Build history of the part. All positions in model axes, mm. Round coordinates to 2 decimals unless told otherwise and drop trailing zeros. Loops run counter-clockwise (first coordinate to the right, second up) from the corner with the lowest first, then second, coordinate; pieces in that order, holes last.
from build123d import *

# Parameters (mm, degrees)
SKETCH1_R           = 2.5
BOSS_EXTRUDE1_DEPTH = 20
SKETCH2_R           = 1.5
CUT_EXTRUDE1_DEPTH  = 5
FILLET1_R           = 0.5


with BuildPart() as part:
    # Sketch1 → Boss-Extrude1 (new body)
    with BuildSketch(Plane(origin=(0, 0, 0), x_dir=(1, 0, 0), z_dir=(0, 1, 0))):
        Circle(SKETCH1_R)
    extrude(amount=BOSS_EXTRUDE1_DEPTH)

    # Sketch2 → Cut-Extrude1 (cut, symmetric)
    with BuildSketch(Plane(origin=(0, 0, 0), x_dir=(0, 0, -1), z_dir=(1, 0, 0))):
        with Locations((0, 17.5)):
            Circle(SKETCH2_R)
        with Locations((0, 2.5)):
            Circle(SKETCH2_R)
    extrude(amount=CUT_EXTRUDE1_DEPTH, both=True, mode=Mode.SUBTRACT)

    # Fillet1
    fillet1_edges = [part.edges().sort_by_distance(p)[0] for p in [
        (-2.5, 0, 0),
        (-2.5, 20, 0),
    ]]
    fillet(fillet1_edges, radius=FILLET1_R)


solid = part.part
(1) Pull direction Z, two halves, no side cores. Call faces 1 (the face through (-2.5, 9.9, -0.1)), 2 (the face through (0.03, 2.57, 1.5)), 3 (the face through (0, 20, 0)): +Z half, -Z half, draft (parallel to the pull), parting line (faces both ways), or undercut.
Responses:
face 1: parting line
face 2: undercut
face 3: draft
(2) Slice it at A-A on z = 0. List the corners of the cut face in (x, y), plus the area to 3 significant figures.
Responses:
outline: (-2.5, 0.5) arc R0.5 ccw to (-2, 0) - (2, 0) arc R0.5 ccw to (2.5, 0.5) - (2.5, 1) - (-2.5, 1) - close; (-2.5, 4) - (2.5, 4) - (2.5, 16) - (-2.5, 16) - close; (-2.5, 19) - (2.5, 19) - (2.5, 19.5) arc R0.5 ccw to (2, 20) - (-2, 20) arc R0.5 ccw to (-2.5, 19.5) - close
area: 69.8 mm2
(3) Pin check, flat tips, straight feed: P1, Ø2, axis at y = 10.5, z = -2, coming from the -X side; P2, Ø2, axis at y = 3, z = -0.5, coming from the -X side. Stop position of each tip, or through.
Responses:
P1: stops at x = -2.29
P2: stops at x = -2.48
(4) Probe line 1 (Y direction, x = -0.75, z = 0); line 2 (Y direction, x = -2, z = 0.55); line 3 (X direction, y = 4.5, z = 1.5). List the from-to ranges inside material, lowest first.
Responses:
line 1: y = 0 to 1, 4 to 16, 19 to 20
line 2: y = 0.01 to 1.1, 3.9 to 16.1, 18.9 to 19.99
line 3: x = -2 to 2
(5) Slice it at C-C on y = 12.75. List the corners of the cut face in (x, z), plus the area to 3 significant figures.
Responses:
outline: circle Ø5 at (0, 0)
area: 19.6 mm2
(6) Slice it at D-D on x = 0.6. Count the separate pieces of the cut face and the enclosed holes in it, plus the area to 3 significant figures.
Responses:
separate pieces: 1
enclosed holes: 2
area: 82.7 mm2
(7) Slice it at B-B on y = 2.5. List the corners of the cut face in (x, z), plus the area to 3 significant figures.
Responses:
outline: (-2, -1.5) arc R2.5 ccw to (2, -1.5) - close; (-2, 1.5) - (2, 1.5) arc R2.5 ccw to start
area: 5.59 mm2
